from build123d import *

# Parameters (mm, degrees)
SKETCH_R      = 5
SKETCH_R_2    = 1.5
PAD_DEPTH     = 10
SKETCH001_R   = 6
SKETCH001_R_2 = 1.5
PAD001_DEPTH  = 1
SKETCH002_R   = 6
SKETCH002_R_2 = 1.5
PAD002_DEPTH  = 1


with BuildPart() as part:
    # Sketch → Pad (new body)
    with BuildSketch(Plane.XY):
        Circle(SKETCH_R)
        Circle(SKETCH_R_2, mode=Mode.SUBTRACT)
    extrude(amount=PAD_DEPTH)

    # Sketch001 (on Face4 of Pad) → Pad001 (join)
    with BuildSketch(Plane.XY.offset(10)):
        Circle(SKETCH001_R)
        Circle(SKETCH001_R_2, mode=Mode.SUBTRACT)
    extrude(amount=PAD001_DEPTH)

    # Sketch002 (on Face2 of Pad001) → Pad002 (join)
    with BuildSketch(Plane(origin=(0, 0, 0), x_dir=(1, 0, 0), z_dir=(0, 0, -1))):
        Circle(SKETCH002_R)
        Circle(SKETCH002_R_2, mode=Mode.SUBTRACT)
    extrude(amount=PAD002_DEPTH)


solid = part.part
Part model, mm, in its own coordinate system. A direction names the side the tool comes from. Give positions to 0.01 mm unless a question says otherwise; leave off trailing zeros. Write each loop counter-clockwise with the first axis right and the second up, starting at its lowest first coordinate (ties: lowest second). Pieces come first, ordered by that corner, then holes.
1) Cut at C-C on z = 3.5. Write the cut outline in (x, y).
Resolved:
outline: circle Ø10 at (0, 0); hole circle Ø3 at (0, 0)
2) Two-plate mould, pull along Y, no slides. Class faces 1 (the face through (-5.994, -0.264, -0.493)), 2 (the face through (1.2, 1.2, -1)), 3 (the face through (-1.5, -0.07, 5.08)): released by +Y, released by -Y, zero draft, split by the parting line, or undercut.
Resolved:
face 1: split by the parting line
face 2: zero draft
face 3: undercut
3) Pin check, flat tips, straight feed: pin 1 (1 mm diameter, centred on y = -4.5, z = 3.5, fed in from -X); pin 2 (1.5 mm diameter, centred on y = 2, z = 7.5, fed in from -X); pin 3 (3 mm diameter, centred on x = -2, z = 2, fed in from +Y). Stop position of each tip, or through.
Resolved:
pin 1: stops at x = -3
pin 2: stops at x = -4.84
pin 3: stops at y = 4.97
4) Cut at A-A on x = 0. Write the cut outline in (y, z), then the cut area to 3 significant figures.
Resolved:
outline: (-6, -1) - (-1.5, -1) - (-1.5, 11) - (-6, 11) - (-6, 10) - (-5, 10) - (-5, 0) - (-6, 0) - close; (1.5, -1) - (6, -1) - (6, 0) - (5, 0) - (5, 10) - (6, 10) - (6, 11) - (1.5, 11) - close
area: 88.0 mm2
5) Which spindle directions (+Z, -Z, +X, -X, +Y, -Y) get a long thin tool onto all of the face, cutting with end or side? Do faces 4 (the face through (-4, -4, 0)), 5 (the face through (1.2, -1.2, 11)). Say none if no direction does.
Resolved:
face 4: none
face 5: +Z, +X, -X, +Y, -Y
6) Probe L1, parallel to Z at x = -4.25, y = 2.75; L2, parallel to Y at x = 0, z = 3.75; L3, parallel to Y at x = -1, z = 9.25. List the from-to ranges inside material, lowest first.
Resolved:
L1: z = -1 to 0, 10 to 11
L2: y = -5 to -1.5, 1.5 to 5
L3: y = -4.9 to -1.12, 1.12 to 4.9
7) Cut at D-D on y = -2. Write the cut outline in (x, z).
Resolved:
outline: (-5.66, -1) - (5.66, -1) - (5.66, 0) - (4.58, 0) - (4.58, 10) - (5.66, 10) - (5.66, 11) - (-5.66, 11) - (-5.66, 10) - (-4.58, 10) - (-4.58, 0) - (-5.66, 0) - close
